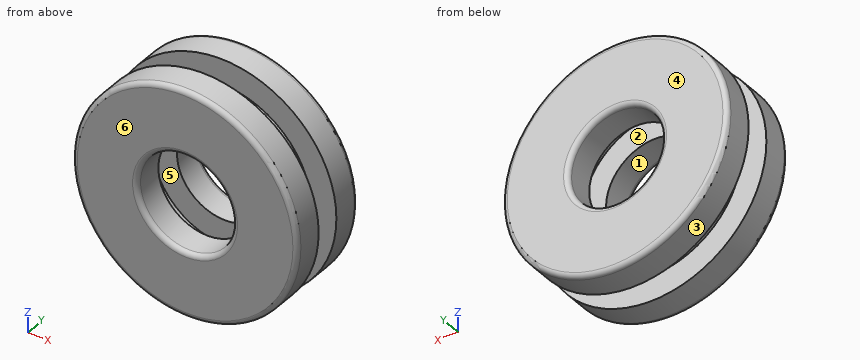
```python
from build123d import *


with BuildPart() as part:
    # Эскиз1 → Повернуть1 (revolve)
    with BuildSketch(Plane.XY):
        with BuildLine():
            Line((5.1, 3.166666667), (7.666666667, 3.166666667))
            Line((7.666666667, 3.166666667), (7.666666667, 5.833333333))
            Line((7.666666667, 5.833333333), (5, 5.833333333))
            Line((5, 5.833333333), (5, 8.5))
            ThreePointArc((5, 8.5), (5.146446609, 8.853553391), (5.5, 9))
            Line((5.5, 9), (11.5, 9))
            ThreePointArc((11.5, 9), (11.853553391, 8.853553391), (12, 8.5))
            Line((12, 8.5), (12, 5.833333333))
            Line((12, 5.833333333), (9.333333333, 5.833333333))
            Line((9.333333333, 5.833333333), (9.333333333, 3.166666667))
            Line((9.333333333, 3.166666667), (12, 3.166666667))
            Line((12, 3.166666667), (12, 0.5))
            ThreePointArc((12, 0.5), (11.853553391, 0.146446609), (11.5, 0))
            Line((11.5, 0), (5.6, 0))
            ThreePointArc((5.6, 0), (5.246446609, 0.146446609), (5.1, 0.5))
            Line((5.1, 0.5), (5.1, 3.166666667))
        make_face()
    revolve(axis=Axis((0, -1000, 0), (0, 1, 0)))


solid = part.part
```
CAD build for the part. Positions are in the model's coordinates, mm. Face numbers are marked on the shaded views. A direction names the side the tool comes from. Round coordinates to 2 decimals unless told otherwise and drop trailing zeros. Write each loop counter-clockwise with the first axis right and the second up, starting at its lowest first coordinate (ties: lowest second). Pieces come first, ordered by that corner, then holes. Notation, with made-up numbers: M -17.75,-0.5 L 31.25,-0.5 A27 ccw 31.25,26.5 Z; hole C -20.75,-39.5 d1. An arc over 180 degrees is marked long. One line per question, with ' | ' between items.
1. Cut at D-D on y = 1. Write the cut outline in (x, z).
Working result:
outline: C 0,0 d24; hole C 0,0 d10.2
2. Mould opens along Y. For the marked faces 4, 5 and 6 say: pulls with the +Y half, pulls with the -Y half, needs draft (parallel to the pull), parting line crosses it, or undercut.
Working result:
face 4: pulls with the +Y half | face 5: undercut | face 6: pulls with the -Y half
3. Which spindle directions (+Z, -Z, +X, -X, +Y, -Y) get a long thin tool onto all of the face, cutting with end or side? Do the marked faces 1, 2 and 3. Say none if no direction does.
Working result:
face 1: -Y | face 2: none | face 3: +Y, -Y
4. Cut at C-C on y = 7.25. Write the cut outline in (x, z), and give its area (3 significant figures).
Working result:
outline: C 0,0 d24; hole C 0,0 d10 | area: 374 mm2
5. Pin check, flat tips, straight feed: pin 1 Ø6 at (x, z) = (8, 9.5) entering from +Y; pin 2 Ø2 at (x, y) = (-4.5, 7) entering from -Z; pin 3 Ø2 at (x, y) = (7, 1.5) entering from +Z; pin 4 Ø1.5 at (x, y) = (-1, 8) entering from -Z. Stop position of each tip, or through.
Working result:
pin 1: y = 9 | pin 2: z = -11.48 | pin 3: z = 10.39 | pin 4: z = -12
6. Probe L1, parallel to X at y = 7.7, z = 0; L2, parallel to Z at x = 0, y = 5; L3, parallel to Y at x = -6, z = -8. List the from-to ranges inside material, lowest first. Write a range as from..to.
Working result:
L1: -12..-5, 5..12 | L2: -9.33..-7.67, 7.67..9.33 | L3: 0..3.17, 5.83..9
